Source: CAD feature listing. Evaluate the final solid. Frame: model axes, mm. Face numbers are marked on the shaded views. A direction names the side the tool comes from. Round coordinates to 2 decimals unless told otherwise and drop trailing zeros. Loops run counter-clockwise (first coordinate to the right, second up) from the corner with the lowest first, then second, coordinate; pieces in that order, holes last. Notation, with made-up numbers: M -16,-38 L -5,-38 A23 ccw -5,-21 Z; hole C 84,1 d2. An arc over 180 degrees is marked long. One line per item, written item: value.
from build123d import *

# Parameters (mm, degrees)
SKETCH1_W                    = 50.8
SKETCH1_H                    = 50.8
SKETCH1_W_2                  = 38.1
SKETCH1_H_2                  = 38.1
BOSS_EXTRUDE1_DEPTH          = 178
SKETCH2_W                    = 44.8
SKETCH2_H                    = 44.8
SKETCH2_W_2                  = 38.1
SKETCH2_H_2                  = 38.1
CUT_EXTRUDE1_DEPTH           = 20
SKETCH3_W                    = 46.8
SKETCH3_H                    = 124.475000116
CUT_EXTRUDE2_DEPTH           = 47.625
SKETCH4_W                    = 50.8
SKETCH4_H                    = 3.175
CUT_EXTRUDE3_DEPTH           = 3.175
SKETCH5_W                    = 3.175
SKETCH5_H                    = 3.175
CUT_EXTRUDE4_DEPTH           = 192.951243809
CUT_EXTRUDE5_DEPTH           = 1
SKETCH7_W                    = 46.8
SKETCH7_H                    = 3.175
CUT_EXTRUDE6_DEPTH           = 1
FILLET1_R                    = 1.5875
CUT_EXTRUDE7_DEPTH           = 2.34442
M1_2X0_25_TAPPED_HOLE1_D     = 0.95
M1_2X0_25_TAPPED_HOLE1_DEPTH = 2.9997
M1_2X0_25_TAPPED_HOLE1_TIP   = 0.285408794
BOSS_EXTRUDE2_REACH          = 193.689
CUT_EXTRUDE8_REACH           = 193.951
SKETCH15_W                   = 30
SKETCH15_H                   = 6.8
FILLET2_R                    = 1.5875
LPATTERN1_COUNT              = 2
LPATTERN1_PITCH              = 20.8


with BuildPart() as part:
    # Sketch1 → Boss-Extrude1 (new body)
    with BuildSketch(Plane(origin=(0, 0, 0), x_dir=(1, 0, 0), z_dir=(0, 1, 0))):
        with Locations((25.4, 25.4)):
            Rectangle(SKETCH1_W, SKETCH1_H)
        with Locations((25.4, 25.4)):
            Rectangle(SKETCH1_W_2, SKETCH1_H_2, mode=Mode.SUBTRACT)
    extrude(amount=BOSS_EXTRUDE1_DEPTH)

    # Sketch2 → Cut-Extrude1 (cut)
    with BuildSketch(Plane.XZ):
        with Locations((25.4, -25.4)):
            Rectangle(SKETCH2_W, SKETCH2_H)
        with Locations((25.4, -25.4)):
            Rectangle(SKETCH2_W_2, SKETCH2_H_2, mode=Mode.SUBTRACT)
    extrude(amount=-CUT_EXTRUDE1_DEPTH, mode=Mode.SUBTRACT)

    # Sketch3 → Cut-Extrude2 (cut)
    with BuildSketch(Plane.XY):
        with Locations((25.4, 109.412499942)):
            Rectangle(SKETCH3_W, SKETCH3_H)
    extrude(amount=-CUT_EXTRUDE2_DEPTH, mode=Mode.SUBTRACT)

    # Sketch4 → Cut-Extrude3 (cut)
    with BuildSketch(Plane.XY):
        with Locations((25.4, 25.5875)):
            Rectangle(SKETCH4_W, SKETCH4_H)
        with Locations((25.4, 38.5875)):
            Rectangle(SKETCH4_W, SKETCH4_H)
    cut_extrude3 = extrude(amount=-CUT_EXTRUDE3_DEPTH, mode=Mode.SUBTRACT)

    # Sketch5 → Cut-Extrude4 (cut, through all)
    with BuildSketch(Plane.XY):
        with Locations((1.5875, 38.5875)):
            Rectangle(SKETCH5_W, SKETCH5_H)
        with Locations((1.5875, 25.5875)):
            Rectangle(SKETCH5_W, SKETCH5_H)
    cut_extrude4 = extrude(amount=-CUT_EXTRUDE4_DEPTH, mode=Mode.SUBTRACT)

    # Sketch6 → Cut-Extrude5 (cut)
    with BuildSketch(Plane.ZY):
        with BuildLine():
            Line((-32.4, 175), (-18.4, 175))
            ThreePointArc((-18.4, 175), (-17.4, 174), (-18.4, 173))
            Line((-18.4, 173), (-32.4, 173))
            ThreePointArc((-32.4, 173), (-33.4, 174), (-32.4, 175))
        make_face()
        with BuildLine():
            Line((-32.4, 171.5), (-18.4, 171.5))
            ThreePointArc((-18.4, 171.5), (-17.4, 170.5), (-18.4, 169.5))
            Line((-18.4, 169.5), (-32.4, 169.5))
            ThreePointArc((-32.4, 169.5), (-33.4, 170.5), (-32.4, 171.5))
        make_face()
        with BuildLine():
            Line((-32.4, 168), (-18.4, 168))
            ThreePointArc((-18.4, 168), (-17.4, 167), (-18.4, 166))
            Line((-18.4, 166), (-32.4, 166))
            ThreePointArc((-32.4, 166), (-33.4, 167), (-32.4, 168))
        make_face()
    cut_extrude5 = extrude(amount=-CUT_EXTRUDE5_DEPTH, mode=Mode.SUBTRACT)

    # Mirror1: Cut-Extrude3 across plane
    add(cut_extrude3.mirror(Plane.XY.offset(-25.4)), mode=Mode.SUBTRACT)

    # Mirror2: Cut-Extrude4, Cut-Extrude5 across plane
    add(cut_extrude4.mirror(Plane.ZY.offset(-25.4)), mode=Mode.SUBTRACT)
    add(cut_extrude5.mirror(Plane.ZY.offset(-25.4)), mode=Mode.SUBTRACT)

    # Sketch7 → Cut-Extrude6 (cut)
    with BuildSketch(Plane.XY):
        with Locations((25.4, 173.2375)):
            Rectangle(SKETCH7_W, SKETCH7_H)
        with Locations((25.4, 45.587499884)):
            Rectangle(SKETCH7_W, SKETCH7_H)
    extrude(amount=-CUT_EXTRUDE6_DEPTH, mode=Mode.SUBTRACT)

    # Fillet1
    fillet1_edges = [part.edges().sort_by_distance(p)[0] for p in [
        (47.8, 10, -3),
        (47.8, 10, -47.8),
        (2, 174.825, -0.5),
        (48.8, 174.825, -0.5),
        (3, 10, -47.8),
        (2, 43.999999884, -0.5),
        (3, 10, -3),
        (48.8, 43.999999884, -0.5),
        (2, 47.174999884, -24.3125),
        (2, 171.65, -24.3125),
        (48.8, 171.65, -24.3125),
        (48.8, 47.174999884, -24.3125),
    ]]
    fillet(fillet1_edges, radius=FILLET1_R)

    # Sketch8 → Cut-Extrude7 (cut)
    with BuildSketch(Plane(origin=(0, 178, 0), x_dir=(1, 0, 0), z_dir=(0, 1, 0))):
        with BuildLine():
            Line((4.7625, 49.2125), (46.0375, 49.2125))
            ThreePointArc((46.0375, 49.2125), (48.28256403, 48.28256403), (49.2125, 46.0375))
            Line((49.2125, 46.0375), (49.2125, 4.7625))
            ThreePointArc((49.2125, 4.7625), (48.28256403, 2.51743597), (46.0375, 1.5875))
            Line((46.0375, 1.5875), (4.7625, 1.5875))
            ThreePointArc((4.7625, 1.5875), (2.51743597, 2.51743597), (1.5875, 4.7625))
            Line((1.5875, 4.7625), (1.5875, 46.0375))
            ThreePointArc((1.5875, 46.0375), (2.51743597, 48.28256403), (4.7625, 49.2125))
        make_face()
    extrude(amount=-CUT_EXTRUDE7_DEPTH, mode=Mode.SUBTRACT)

    # M1.2x0.25 Tapped Hole1
    with Locations(Plane.XY.offset(-1)):
        with Locations((3.8415, 172.98375321), (46.95875321, 172.98375321), (3.8415, 45.841499884), (46.95875321, 45.841499884)):
            Hole(M1_2X0_25_TAPPED_HOLE1_D / 2, depth=M1_2X0_25_TAPPED_HOLE1_DEPTH)
            with Locations((0, 0, -(M1_2X0_25_TAPPED_HOLE1_DEPTH + M1_2X0_25_TAPPED_HOLE1_TIP / 2))):  # 118° drill point
                Cone(0, M1_2X0_25_TAPPED_HOLE1_D / 2, M1_2X0_25_TAPPED_HOLE1_TIP, mode=Mode.SUBTRACT)

    # Sketch17 → Boss-Extrude2 (add, up to next)
    with BuildSketch(Plane.XY.offset(-1), mode=Mode.PRIVATE) as boss_extrude2_sk1:
        with BuildLine():
            Line((2, 170.0625), (2, 48.762499884))
            ThreePointArc((2, 48.762499884), (2.464967985, 47.639967869), (3.5875, 47.174999884))
            Line((3.5875, 47.174999884), (5.5875, 47.174999884))
            ThreePointArc((5.5875, 47.174999884), (4.464967985, 47.639967869), (4, 48.762499884))
            Line((4, 48.762499884), (4, 170.0625))
            ThreePointArc((4, 170.0625), (4.464967985, 171.185032015), (5.5875, 171.65))
            Line((5.5875, 171.65), (3.5875, 171.65))
            ThreePointArc((3.5875, 171.65), (2.464967985, 171.185032015), (2, 170.0625))
        make_face()
    boss_extrude2_tool1 = extrude(boss_extrude2_sk1.sketch, amount=-BOSS_EXTRUDE2_REACH, mode=Mode.PRIVATE) - part.part
    add(boss_extrude2_tool1.solids().sort_by_distance((3.00869, 109.4125, -1))[0])

    # Sketch15 → Cut-Extrude8 (cut, up to next)
    with BuildSketch(Plane.ZY, mode=Mode.PRIVATE) as cut_extrude8_sk1:
        with Locations((-25.4, 105)):
            Rectangle(SKETCH15_W, SKETCH15_H)
    cut_extrude8_tool1 = extrude(cut_extrude8_sk1.sketch, amount=-CUT_EXTRUDE8_REACH, mode=Mode.PRIVATE) & part.part
    # Sketch15 → Cut-Extrude8 (cut, up to next)
    with BuildSketch(Plane.ZY, mode=Mode.PRIVATE) as cut_extrude8_sk2:
        with Locations((-25.4, 125.8)):
            Rectangle(SKETCH15_W, SKETCH15_H)
    cut_extrude8_tool2 = extrude(cut_extrude8_sk2.sketch, amount=-CUT_EXTRUDE8_REACH, mode=Mode.PRIVATE) & part.part
    add(cut_extrude8_tool1.solids().sort_by_distance((0, 105, -25.4))[0], mode=Mode.SUBTRACT)
    add(cut_extrude8_tool2.solids().sort_by_distance((0, 125.8, -25.4))[0], mode=Mode.SUBTRACT)

    # Fillet2
    fillet2_edges = [part.edges().sort_by_distance(p)[0] for p in [
        (2, 101.6, -10.4),
        (2, 108.4, -10.4),
        (2, 108.4, -40.4),
        (2, 101.6, -40.4),
        (2, 122.4, -10.4),
        (2, 129.2, -10.4),
        (2, 129.2, -40.4),
        (2, 122.4, -40.4),
    ]]
    fillet(fillet2_edges, radius=FILLET2_R)

    # Sketch20 → Cut-Revolve1 (revolve, cut)
    with BuildSketch(Plane(origin=(0, 125.8, 0), x_dir=(1, 0, 0), z_dir=(0, 1, 0))):
        with BuildLine():
            Line((-16.55, 25.4), (2.5, 25.4))
            ThreePointArc((2.5, 25.4), (-16.55, 6.35), (-35.6, 25.4))
            Line((-35.6, 25.4), (-16.55, 25.4))
        make_face()
    cut_revolve1 = revolve(axis=Axis((-16.55, 125.8, -25.4), (1, 0, 0)), mode=Mode.SUBTRACT)

    # LPattern1: Cut-Revolve1 ×2
    with Locations(*[(0, -i * LPATTERN1_PITCH, 0) for i in range(1, LPATTERN1_COUNT)]):
        add(cut_revolve1, mode=Mode.SUBTRACT)


solid = part.part
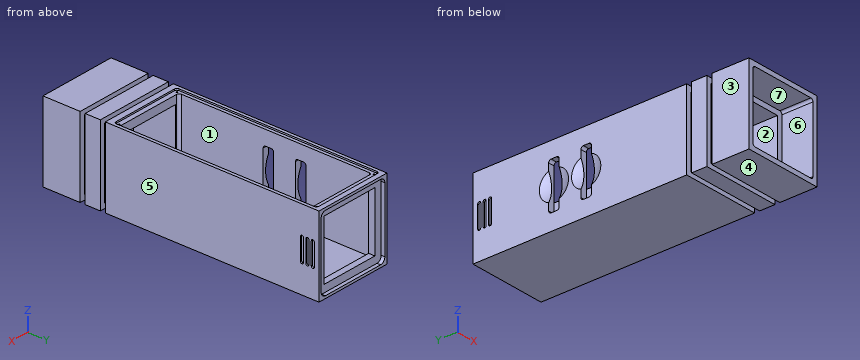
1. Reachability of the marked faces 1, 2 and 3 from +Z, -Z, +X, -X, +Y, -Y: full face, straight path, thin tool, end or side. Return the list, or none.
Report:
face 1: +Z
face 2: +Y, -Y
face 3: +Z, -Z, -X, +Y, -Y
2. Section query B-B (x = 39). Count the separate pieces of the cut face and the enclosed holes in it, and give its area (3 significant figures).
Report:
separate pieces: 3
enclosed holes: 0
area: 872 mm2
3. Section query A-A (y = 73). Return the cut outline in (x, z) (3 decimals).
Report:
outline: M 0,-50.8 L 50.8,-50.8 L 50.8,0 L 48.8,0 L 48.8,-47.625 L 4,-47.625 L 4,-1 L 2,-1 L 2,0 L 0,0 Z
4. Pin query (flat end, axial travel): pin 1 (4 mm diameter, centred on y = 142.5, z = -31, fed in from -X); pin 2 (1.1 mm diameter, centred on x = 3, y = 126.5, fed in from +Z); pin 3 (12 mm diameter, centred on x = 34, y = 101.5, fed in from +Z) (3 decimals); pin 4 (1.2 mm diameter, centred on y = 174, z = -29, fed in from +X). Return the tip coordinate at first contact, or that it passes through.
Report:
pin 1: stops at x = 0
pin 2: stops at z = -1
pin 3: stops at z = -47.625
pin 4: stops at x = 49.8
5. Pull-direction query (Z, two-part tool) for the marked faces 4, 5, 6 and 7; classes: released by +Z, released by -Z, zero draft, split by the parting line, or undercut.
Report:
face 4: released by -Z
face 5: zero draft
face 6: undercut
face 7: undercut
6. Ray query, line 1 (Y direction, x = 13.5, z = -47) (3 decimals); line 2 (X direction, y = 18, z = -20.5); line 3 (Z direction, x = 22.5, y = 43.5). Return the intervals inside material, ascending. Write a range as [from, to].
Report:
line 1: y = [20, 47.175], [171.65, 175.656]
line 2: x = [0, 3], [47.8, 50.8]
line 3: z = [-50.8, -44.45], [-6.35, 0]
